Work out the finished part from the listing and answer in its coordinate system (mm). Round coordinates to 2 decimals unless told otherwise and drop trailing zeros. Order: outer loops, then holes, each group sorted by start corner. A loop starts at its lowest first (then second) coordinate and runs counter-clockwise, first axis right, second up. Notation, with made-up numbers: (-28, -30.5) - (-14, -30.5) arc R8 ccw to (-14, -21.5) - close; hole circle Ø11 at (17.25, 37.5). An arc over 180 degrees is marked (long way). Use one line per item in the form item = value. Start each with the question number.
Q1. The part is cut by section C-C on x = -14. Determine the outline of the cut face in (y, z), plus the area to 3 significant figures.
Q2. The part is cut by section B-B on z = 0. Determine the outline of the cut face in (x, y), plus the area to 3 significant figures.
Q3. The part is cut by section D-D on y = 0.55. State how many separate pieces and enclosed holes the cut face has, plus the area to 3 significant figures.
Q4. The part is cut by section A-A on x = 8.5. Determine the outline of the cut face in (y, z), plus the area to 3 significant figures.
Q5. Find the intervals of material crossed by line 1 (X direction, y = 0.3, z = 0); line 2 (Z direction, x = -14, y = 0.2); line 3 (X direction, y = 0.45, z = -1.5), in increasing order. Write a range as [from, to].
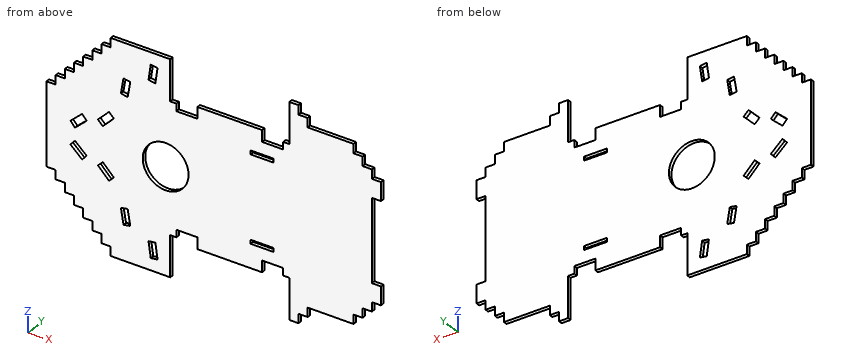
from build123d import *

# Parameters (mm, degrees)
SKETCH_5_R      = 5
SKETCH_5_W      = 5
SKETCH_5_H      = 0.85
EXTRUDE_1_DEPTH = 0.8


with BuildPart() as part:
    # 스케치5 → 보스-돌출1 (new body)
    with BuildSketch(Plane(origin=(0, 0, 0), x_dir=(1, 0, 0), z_dir=(0, 1, 0))):
        Polygon((-13, -23), (-13, -14.1), (-11.65, -14.1), (-11.65, -12.5), (-7.05, -12.5), (-7.05, -14.1), (-7.05, -15), (7.05, -15), (7.05, -14.1), (7.05, -12.5), (11.65, -12.5), (11.65, -14.1), (13, -14.1), (13, -23), (15, -23), (15, -21), (17, -21), (17, -19), (27, -19), (27, -17), (29, -17), (29, -15), (31, -15), (31, -13), (33, -13), (33, -9), (31, -9), (31, 9), (33, 9), (33, 13), (31, 13), (31, 15), (29, 15), (29, 17), (27, 17), (27, 19), (17, 19), (17, 21), (15, 21), (15, 23), (13, 23), (13, 14.1), (11.65, 14.1), (11.65, 12.5), (7.05, 12.5), (7.05, 14.1), (7.05, 15), (-7.05, 15), (-7.05, 14.1), (-7.05, 12.5), (-11.65, 12.5), (-11.65, 14.1), (-13, 14.1), (-13, 23), (-26, 23), (-26, 21), (-28, 21), (-28, 19), (-30, 19), (-30, 17), (-32, 17), (-32, 15), (-34, 15), (-34, 13), (-36, 13), (-36, 11), (-38, 11), (-38, 9), (-40, 9), (-40, -9), (-38, -9), (-38, -11), (-36, -11), (-36, -13), (-34, -13), (-34, -15), (-32, -15), (-32, -17), (-30, -17), (-30, -19), (-28, -19), (-28, -21), (-26, -21), (-26, -23), align=None)
        with Locations((-14, 0)):
            Circle(SKETCH_5_R, mode=Mode.SUBTRACT)
        Polygon((-17.728524487, -17.009831185), (-17.241222705, -20.415141299), (-15.756349109, -20.202655057), (-16.243650891, -16.797344943), align=None, mode=Mode.SUBTRACT)
        Polygon((-23.763263852, -12.051103665), (-23.19560882, -15.443944328), (-21.716172484, -15.196420332), (-22.283827516, -11.803579668), align=None, mode=Mode.SUBTRACT)
        Polygon((-28.776184385, -4.834516937), (-26.354359033, -7.277540056), (-25.289087324, -6.22151156), (-27.710912676, -3.77848844), align=None, mode=Mode.SUBTRACT)
        Polygon((-32.230719309, -4.802671603), (-34.781815362, -2.494965181), (-33.775548026, -1.382568646), (-31.224451974, -3.690275068), align=None, mode=Mode.SUBTRACT)
        Polygon((-17.241222705, 20.415141299), (-15.756349109, 20.202655057), (-16.243650891, 16.797344943), (-17.728524487, 17.009831185), align=None, mode=Mode.SUBTRACT)
        Polygon((-23.19560882, 15.443944328), (-21.716172484, 15.196420332), (-22.283827516, 11.803579668), (-23.763263852, 12.051103665), align=None, mode=Mode.SUBTRACT)
        Polygon((-26.354359033, 7.277540056), (-25.289087324, 6.22151156), (-27.710912676, 3.77848844), (-28.776184385, 4.834516937), align=None, mode=Mode.SUBTRACT)
        Polygon((-34.781815362, 2.494965181), (-33.775548026, 1.382568646), (-31.224451974, 3.690275068), (-32.230719309, 4.802671603), align=None, mode=Mode.SUBTRACT)
        with Locations((7.05, 9.425)):
            Rectangle(SKETCH_5_W, SKETCH_5_H, mode=Mode.SUBTRACT)
        with Locations((7.05, -9.425)):
            Rectangle(SKETCH_5_W, SKETCH_5_H, mode=Mode.SUBTRACT)
    extrude(amount=EXTRUDE_1_DEPTH)


solid = part.part
Found:
q1.outline = (0, -23) - (0.8, -23) - (0.8, -5) - (0, -5) - close; (0, 5) - (0.8, 5) - (0.8, 23) - (0, 23) - close
q1.area = 28.8 mm²
q2.outline = (-40, 0) - (-19, 0) - (-19, 0.8) - (-40, 0.8) - close; (-9, 0) - (31, 0) - (31, 0.8) - (-9, 0.8) - close
q2.area = 48.8 mm²
q3.separate_pieces = 1
q3.enclosed_holes = 11
q3.area = 2,320 mm²
q4.outline = (0, -12.5) - (0.8, -12.5) - (0.8, -9.85) - (0, -9.85) - close; (0, -9) - (0.8, -9) - (0.8, 9) - (0, 9) - close; (0, 9.85) - (0.8, 9.85) - (0.8, 12.5) - (0, 12.5) - close
q4.area = 18.6 mm²
q5.line_1 = [-40, -19], [-9, 31]
q5.line_2 = [-23, -5], [5, 23]
q5.line_3 = [-40, -33.88], [-33.65, -18.77], [-9.23, 31]
